Could you check a few things on this model? Use its own coordinates, in mm. Give positions to 0.01 mm unless a question says otherwise; leave off trailing zeros. Order: outer loops, then holes, each group sorted by start corner. A loop starts at its lowest first (then second) coordinate and runs counter-clockwise, first axis right, second up.
from build123d import *

# Parameters (mm, degrees)
SKETCH_W        = 15
SKETCH_H        = 15
SKETCH_W_2      = 12
SKETCH_H_2      = 12
PAD_DEPTH       = 500
SKETCH001_R     = 2
POCKET_DEPTH    = 5
SKETCH002_R     = 2
POCKET001_DEPTH = 30


with BuildPart() as part:
    # Sketch → Pad (new body)
    with BuildSketch(Plane.XY):
        Rectangle(SKETCH_W, SKETCH_H)
        Rectangle(SKETCH_W_2, SKETCH_H_2, mode=Mode.SUBTRACT)
    extrude(amount=PAD_DEPTH)

    # Sketch001 → Pocket (cut)
    with BuildSketch(Plane.XZ.offset(7.5)):
        with Locations((0, 195.4891)):
            Circle(SKETCH001_R)
        with Locations((0, 96)):
            Circle(SKETCH001_R)
        with Locations((0, 294.9782)):
            Circle(SKETCH001_R)
        with Locations((0, 394.4673)):
            Circle(SKETCH001_R)
    extrude(amount=-POCKET_DEPTH, mode=Mode.SUBTRACT)

    # Sketch002 → Pocket001 (cut)
    with BuildSketch(Plane(origin=(-7.5, 0, 0), x_dir=(0, -1, 0), z_dir=(-1, 0, 0))):
        with Locations((0, 375)):
            Circle(SKETCH002_R)
        with Locations((0, 125)):
            Circle(SKETCH002_R)
    extrude(amount=-POCKET001_DEPTH, mode=Mode.SUBTRACT)


solid = part.part
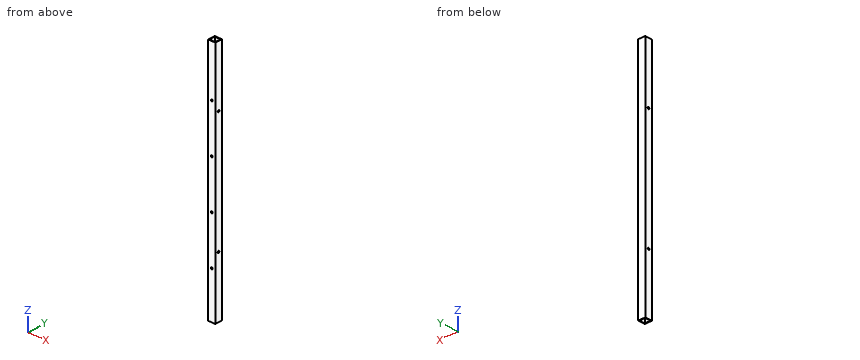
Item 1: Imagine slicing it at A-A on z = 176. List the corners of the cut face in (x, y) for me.
Findings:
outline: (-7.5, -7.5) - (7.5, -7.5) - (7.5, 7.5) - (-7.5, 7.5) - close; hole (-6, -6) - (6, -6) - (6, 6) - (-6, 6) - close
Item 2: Please list where these lines run through material, in increasing order: line 1 along Z through (x, y) = (0, -6.7); line 2 along X through (y, z) = (-4, 34).
Findings:
line 1: z = 0 to 94, 98 to 193.49, 197.49 to 292.98, 296.98 to 392.47, 396.47 to 500
line 2: x = -7.5 to -6, 6 to 7.5
Item 3: For pin 1 (6.5 mm diameter, centred on x = 0, z = 394.47, fed in from -Y); pin 2 (3 mm diameter, centred on x = 0, z = 294.98, fed in from -Y), each with a flat end and sliding along its axis, tell me the tip position at first contact or that it passes through.
Findings:
pin 1: stops at y = -7.5
pin 2: stops at y = 6
